Autodesk Inventor part; units mm, degrees
ref_plane "Work Plane1" through (6.5, 7.3309, 55.4325) normal (0, 0, 1) x (1, 0, 0)
ref_plane "Work Plane2" through (0, 7.5, 60) normal (0, 1, 0) x (-1, 0, 0)
ref_plane "YZ Plane" through (0, 0, 0) normal (1, 0, 0) x (0, 1, 0)
sketch "Sketch1" plane through (0, 0, 0) normal (0, 0, 1) x (1, 0, 0)
  line L0 (-30, 7.5) -> (30, 7.5)
  line L1 (30, 7.5) -> (30, -7.5)
  line L2 (30, -7.5) -> (-30, -7.5)
  line L3 (-30, -7.5) -> (-30, 7.5)
  line L4 (-30, 7.5) -> (30, -7.5) construction
  line L5 (30, 7.5) -> (-30, -7.5) construction
  point P0 (0, 0)
  dimension "d0" = 60
  dimension "d1" = 15
extrude "Extrusion1" add sketch "Sketch1" along normal blind 60
sketch "Sketch3" plane through (-30, 7.5, 0) normal (0, 1, 0) x (1, 0, 0)
  circle A0 centre (30, -30) radius 26.25
  line L0 (60, 0) -> (0, 0)
  line L1 (60, -60) -> (0, -60)
  line L2 (60, 0) -> (60, -60)
  line L3 (36.5, -55.4325) -> (36, -60)
  line L4 (36, -60) -> (24, -60)
  line L5 (24, -60) -> (23.5, -55.4325)
  point P0 (30, 0)
  point P1 (31.6579, -56.1976)
  point P2 (30, 0)
  point P3 (60, -30)
  point P4 (30, -60)
  point P5 (24, -60)
  dimension "d14" = 52.5
  dimension "d16" = 30
  dimension "d17" = 12
  dimension "d18" = 13
  dimension "d26" = 25.4325
extrude "Extrusion3" cut sketch "Sketch3" against normal blind 15
sketch "Sketch4" plane through (0, 0, 60) normal (0, 0, 1) x (1, 0, 0)
  circle A0 centre (0, -117.5) radius 125
  line L0 (-26.25, 7.5) -> (26.25, 7.5)
  point P0 (0, 0)
  point P1 (-6.5, 7.5)
  point P2 (6.5, 7.5)
  dimension "d19" = 250
extrude "Extrusion4" cut sketch "Sketch4" against normal through all keep common part
sketch "Sketch6" plane through (0, 0, 60) normal (0, 0, 1) x (1, 0, 0)
  arc A0 (0, 4.5) -> (-6, -3.5) centre (6.6, -6.7) ccw
  line L0 (0, 0) -> (0, -5.1929) construction
  arc A1 (6, -3.5) -> (0, 4.5) centre (-6.6, -6.7) ccw
  line L1 (-6, -3.5) -> (-6, 7.3559)
  line L2 (6, 7.3559) -> (6, -3.5)
  line L3 (-6, 7.3559) -> (6, 7.3559)
  line L4 (26.25, -7.5) -> (-26.25, -7.5) construction
  line L5 (-6, -7.5) -> (-6, 7.3559) construction
  point P0 (6.5, -7.5)
  point P1 (-6.5, -7.5)
  dimension "d27" = 13
  dimension "d31" = 12
  dimension "d35" = 4
ref_plane "Work Plane1" through (6.5, 7.3309, 55.4325) normal (0, 0, 1) x (1, 0, 0)
sketch "Sketch7" plane through (6.5, 7.3309, 55.4325) normal (0, 0, 1) x (1, 0, 0)
  line L0 (19.75, -14.8309) -> (-32.75, -14.8309) construction
  line L1 (-6.5, -14.8309) -> (-6.5, -0.6329) construction
  line L2 (-13, 0) -> (-13, -14.8309) construction
  line L3 (0, 0) -> (0, -14.8309) construction
  line L4 (-6.5, -14.8309) -> (-6.5, 0.8827) construction
  arc A0 (-6.5, -0.8309) -> (-13, -7.8309) centre (-0.8899, -12.5581) ccw
  arc A1 (0, -7.8309) -> (-6.5, -0.8309) centre (-12.1101, -12.5581) ccw
  line L5 (-13, 0) -> (0, 0)
  line L6 (-13, -7.8309) -> (-13, 0)
  line L7 (0, -7.8309) -> (0, 0)
  dimension "d32" = 14
  dimension "d33" = 13
  dimension "d34" = 7
loft "Loft1" add profiles "Sketch7", "Sketch6"
ref_plane "Work Plane2" through (0, 7.5, 60) normal (0, 1, 0) x (-1, 0, 0)
sketch "Sketch8" plane through (0, 7.5, 60) normal (0, 1, 0) x (-1, 0, 0)
  line L0 (22.3834, -56.8) -> (20.7668, -54)
  line L1 (20.7668, -54) -> (22.3834, -51.2)
  line L2 (22.3834, -51.2) -> (25.6166, -51.2)
  line L3 (25.6166, -51.2) -> (27.2332, -54)
  line L4 (27.2332, -54) -> (25.6166, -56.8)
  line L5 (25.6166, -56.8) -> (22.3834, -56.8)
  arc A0 (-6.5, -4.5675) -> (6.5, -4.5675) centre (0, -30) ccw construction
  line L6 (26.8, -7.6166) -> (24, -9.2332)
  line L7 (24, -9.2332) -> (21.2, -7.6166)
  line L8 (21.2, -7.6166) -> (21.2, -4.3834)
  line L9 (21.2, -4.3834) -> (24, -2.7668)
  line L10 (24, -2.7668) -> (26.8, -4.3834)
  line L11 (26.8, -4.3834) -> (26.8, -7.6166)
  line L12 (-22.3834, -3.2) -> (-20.7668, -6)
  line L13 (-20.7668, -6) -> (-22.3834, -8.8)
  line L14 (-22.3834, -8.8) -> (-25.6166, -8.8)
  line L15 (-25.6166, -8.8) -> (-27.2332, -6)
  line L16 (-27.2332, -6) -> (-25.6166, -3.2)
  line L17 (-25.6166, -3.2) -> (-22.3834, -3.2)
  line L18 (-26.8, -52.3834) -> (-24, -50.7668)
  line L19 (-24, -50.7668) -> (-21.2, -52.3834)
  line L20 (-21.2, -52.3834) -> (-21.2, -55.6166)
  line L21 (-21.2, -55.6166) -> (-24, -57.2332)
  line L22 (-24, -57.2332) -> (-26.8, -55.6166)
  line L23 (-26.8, -55.6166) -> (-26.8, -52.3834)
  point P0 (0, -60)
  point P1 (24, -54)
  point P2 (0, -56.25)
  point P3 (0, -30)
  point P4 (24, -6)
  point P5 (-24, -6)
  point P6 (-24, -54)
  dimension "d40" = 24
  dimension "d41" = 5.6
  dimension "d42" = 24
  dimension "d45" = 360
extrude "Extrusion5" cut sketch "Sketch8" against normal blind 5.5
sketch "Sketch9" plane through (0, 7.5, 60) normal (0, 1, 0) x (-1, 0, 0)
  circle A0 centre (24, -54) radius 1.65
  arc A1 (-6.5, -4.5675) -> (6.5, -4.5675) centre (0, -30) ccw construction
  circle A2 centre (24, -6) radius 1.65
  circle A3 centre (-24, -6) radius 1.65
  circle A4 centre (-24, -54) radius 1.65
  point P0 (0, -60)
  point P1 (0, -56.25)
  point P2 (0, -30)
  dimension "d49" = 3.3
  dimension "d50" = 24
  dimension "d51" = 24
  dimension "d54" = 360
extrude "Extrusion6" cut sketch "Sketch9" against normal through all
properties part number "antenna_socket" material "Acetal Resin, Black"
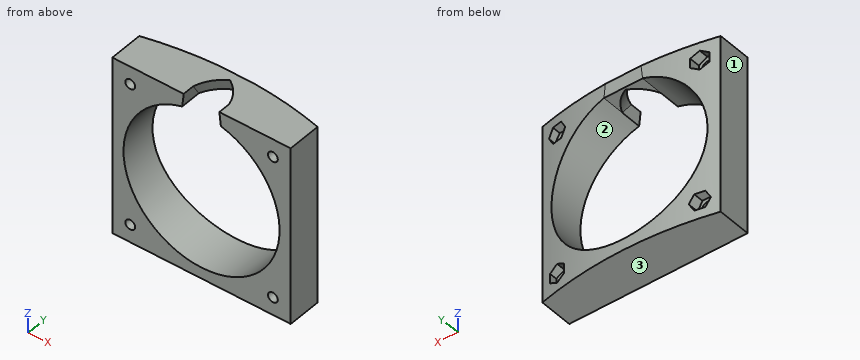
Check sheet for the modelled part. Datum: model origin and axes. Units: mm. Face numbers are marked on the shaded views. Coordinates: 2 decimals unless noted, no trailing zeros. Loops run counter-clockwise (first coordinate to the right, second up) from the corner with the lowest first, then second, coordinate; pieces in that order, holes last.
1) Release check for a two-part mould opening along Z. For the marked faces 1, 2 and 3 record: released by +Z, released by -Z, zero draft, split by the parting line, or undercut.
2) Material ranges on probe 1 along X at (y, z) = (-2.5, 30); probe 2 along Z at (x, y) = (24, -0.75); probe 3 along X at (y, z) = (-6.75, 55.5), recorded low to high.
3) Sectioned sample at C-C (y = -2.25). Count the separate pieces of the cut face and the enclosed holes in it, and give its area (3 significant figures).
4) Sectioned sample at A-A (z = 32). Record the boundary of the cut face in (x, y), and give its area (3 significant figures).
5) Sectioned sample at B-B (z = 42). Record the boundary of the cut face in (x, y).
6) Gauge pin test, flat ends, axial feed: pin 1 (4 mm diameter, centred on x = -24, z = 54, fed in from +Y); pin 2 (12 mm diameter, centred on x = 18.5, z = 42.5, fed in from +Y); pin 3 (2 mm diameter, centred on x = 24, z = 54, fed in from -Y); pin 4 (6 mm diameter, centred on x = -24, z = 4.5, fed in from +Y). Record the tip position at first contact, or that the pin passes through.
Check sheet entries:
1. face 1: zero draft
1. face 2: undercut
1. face 3: released by -Z
2. probe 1: x = -30 to -26.25, 26.25 to 30
2. probe 2: z = 0 to 4.35, 7.65 to 19.37, 40.63 to 52.35, 55.65 to 60
2. probe 3: x = -30 to -24.69, -23.31 to -6.49, 6.49 to 23.31, 24.69 to 30
3. separate pieces: 1
3. enclosed holes: 4
3. area: 1,350 mm2
4. outline: (-30, -7.5) - (-26.17, -7.5) - (-26.17, 4.73) arc R125 ccw to (-30, 3.85) - close; (26.17, -7.5) - (30, -7.5) - (30, 3.85) arc R125 ccw to (26.17, 4.73) - close
4. area: 90.3 mm2
5. outline: (-30, -7.5) - (-23.35, -7.5) - (-23.35, 5.3) arc R125 ccw to (-30, 3.85) - close; (23.35, -7.5) - (30, -7.5) - (30, 3.85) arc R125 ccw to (23.35, 5.3) - close
6. pin 1: stops at y = 2
6. pin 2: stops at y = 6.1
6. pin 3: passes through
6. pin 4: stops at y = 5.72
